CAD build for the part. Positions are in the model's coordinates, mm. Face numbers are marked on the shaded views. A direction names the side the tool comes from. Coordinates: 2 decimals unless noted, no trailing zeros. Loops run counter-clockwise (first coordinate to the right, second up) from the corner with the lowest first, then second, coordinate; pieces in that order, holes last. Notation, with made-up numbers: (59, 72) - (73, 72) arc R29 cw to (73, 94) - close; hole circle Ø7 at (34.25, 35.25). An arc over 180 degrees is marked (long way). Put each result on its own line as item: value.
```python
from build123d import *

# Parameters (mm, degrees)
SKETCH1_R           = 20
BOSS_EXTRUDE1_DEPTH = 12.5
SKETCH2_W           = 25
SKETCH2_H           = 400
BOSS_EXTRUDE2_DEPTH = 100
CUT_EXTRUDE1_REACH  = 705.673
SKETCH3_R           = 7.94
FILLET1_R           = 40


with BuildPart() as part:
    # Sketch1 → Boss-Extrude1 (new, symmetric)
    with BuildSketch(Plane.XY):
        with BuildLine():
            Line((405, -50), (105, -50))
            Line((105, -50), (5, -150))
            Line((5, -150), (5, -350))
            Line((5, -350), (-145, -350))
            Line((-145, -350), (-145, 50))
            Line((-145, 50), (405, 50))
            ThreePointArc((405, 50), (455, 0), (405, -50))
        make_face()
        with Locations((405, 0)):
            Circle(SKETCH1_R, mode=Mode.SUBTRACT)
        with Locations((-20, -70)):
            Circle(SKETCH1_R, mode=Mode.SUBTRACT)
    extrude(amount=BOSS_EXTRUDE1_DEPTH, both=True)

    # Sketch2 → Boss-Extrude2 (add)
    with BuildSketch(Plane.XY.offset(12.5)):
        with Locations((-132.5, -150)):
            Rectangle(SKETCH2_W, SKETCH2_H)
    extrude(amount=BOSS_EXTRUDE2_DEPTH)

    # Sketch3 → Cut-Extrude1 (cut, up to next)
    with BuildSketch(Plane.ZY.offset(145), mode=Mode.PRIVATE) as cut_extrude1_sk1:
        with Locations((87.648409676, 10)):
            Circle(SKETCH3_R)
    cut_extrude1_tool1 = extrude(cut_extrude1_sk1.sketch, amount=-CUT_EXTRUDE1_REACH, mode=Mode.PRIVATE) & part.part
    # Sketch3 → Cut-Extrude1 (cut, up to next)
    with BuildSketch(Plane.ZY.offset(145), mode=Mode.PRIVATE) as cut_extrude1_sk2:
        with Locations((87.648409676, -310)):
            Circle(SKETCH3_R)
    cut_extrude1_tool2 = extrude(cut_extrude1_sk2.sketch, amount=-CUT_EXTRUDE1_REACH, mode=Mode.PRIVATE) & part.part
    add(cut_extrude1_tool1.solids().sort_by_distance((-145, 10, 87.64841))[0], mode=Mode.SUBTRACT)
    add(cut_extrude1_tool2.solids().sort_by_distance((-145, -310, 87.64841))[0], mode=Mode.SUBTRACT)

    # Fillet1
    fillet1_edges = [part.edges().sort_by_distance(p)[0] for p in [
        (-132.5, -350, 112.5),
        (-132.5, 50, 112.5),
    ]]
    fillet(fillet1_edges, radius=FILLET1_R)


solid = part.part
```
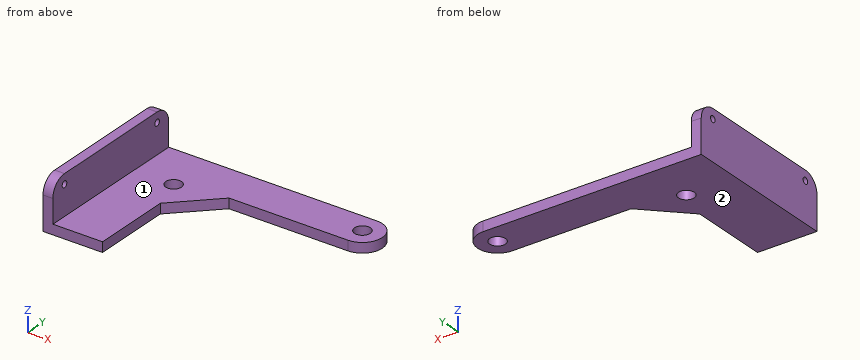
Q1. Pin check, flat tips, straight feed: pin 1 Ø9.5 at (y, z) = (10, 87.65) entering from +X; pin 2 Ø12.5 at (x, z) = (314, 3) entering from -Y; pin 3 Ø20 at (y, z) = (-215, -0.5) entering from +X; pin 4 Ø2 at (y, z) = (-131.5, 18) entering from +X. Stop position of each tip, or through.
Determined:
pin 1: through
pin 2: y = -50
pin 3: x = 5
pin 4: x = -120
Q2. Slice it at A-A, the plane y = -70. Give the cut face in (x, z), then the cut area to 3 significant figures.
Determined:
outline: (-145, -12.5) - (-40, -12.5) - (-40, 12.5) - (-120, 12.5) - (-120, 112.5) - (-145, 112.5) - close; (0, -12.5) - (85, -12.5) - (85, 12.5) - (0, 12.5) - close
area: 7,250 mm2
Q3. Slice it at B-B, the plane z = 86.5. Give the cut face in (x, y).
Determined:
outline: (-145, -347.47) - (-120, -347.47) - (-120, -317.86) - (-145, -317.86) - close; (-145, -302.14) - (-120, -302.14) - (-120, 2.14) - (-145, 2.14) - close; (-145, 17.86) - (-120, 17.86) - (-120, 47.47) - (-145, 47.47) - close
Q4. Tool access for the marked faces 1 and 2: list every direction of +Z, -Z, +X, -X, +Y, -Y with a clear straight run to the whole face (end or side of a thin tool).
Determined:
face 1: +Z, +X, +Y, -Y
face 2: -Z, +X, -X, +Y, -Y
Q5. Slice it at D-D, the plane z = 22.5. Give the cut face in (x, y).
Determined:
outline: (-145, -350) - (-120, -350) - (-120, 50) - (-145, 50) - close
Q6. Slice it at C-C, the plane x = 27.5. Give the cut face in (y, z).
Determined:
outline: (-127.5, -12.5) - (50, -12.5) - (50, 12.5) - (-127.5, 12.5) - close
Q7. Wall check: L1, parallel to Y at x = -20, z = -2; L2, parallel to X at y = -269, z = 81.5; L3, parallel to Y at x = 327, z = 10.5. Give the ranges that are in metal, low to high. Write a range as from..to.
Determined:
L1: -350..-90, -50..50
L2: -145..-120
L3: -50..50
